Build history of the part. All positions in model axes, mm. Round coordinates to 2 decimals unless told otherwise and drop trailing zeros. Loops run counter-clockwise (first coordinate to the right, second up) from the corner with the lowest first, then second, coordinate; pieces in that order, holes last. Notation, with made-up numbers: (-32.5, 8.25) - (2.5, 8.25) arc R18 cw to (2.5, 20.25) - close; hole circle Ø1 at (59.25, -1). An arc over 180 degrees is marked (long way). Use one line per item in the form item = value. Start each with the question number.
Q1. Saw through at B-B (x = -27). Give the cut face in (y, z).
Q2. Drill centre lines: line 1 (Z direction, x = -26.5, y = 0.8); line 2 (X direction, y = 1.55, z = -35). Where is each one in solid material? Low to high.
Q3. Pin check, flat tips, straight feed: pin 1 (8 mm diameter, centred on x = -1.5, z = -128.5, fed in from -Y); pin 2 (1.5 mm diameter, centred on y = 1, z = -205, fed in from -X); pin 3 (1.5 mm diameter, centred on y = 1.5, z = -79, fed in from -X); pin 4 (1.5 mm diameter, centred on x = -37, y = 2, fed in from -Z). Stop position of each tip, or through.
Q4. Saw through at A-A (z = -177.5). Give the cut face in (x, y).
```python
from build123d import *

# Parameters (mm, degrees)
SKETCH1_W           = 35.65
SKETCH1_H           = 204
BOSS_EXTRUDE1_DEPTH = 3
SKETCH2_W           = 12
SKETCH2_H           = 3
SKETCH2_W_2         = 10
BOSS_EXTRUDE2_DEPTH = 3
ESQUISSE1_W         = 10
ESQUISSE1_H         = 3
BOSS_EXTRU_1_DEPTH  = 3
ESQUISSE2_W         = 10
ESQUISSE2_H         = 3
BOSS_EXTRU_2_DEPTH  = 3


with BuildPart() as part:
    # Sketch1 → Boss-Extrude1 (new body)
    with BuildSketch(Plane(origin=(0, 0, 0), x_dir=(1, 0, 0), z_dir=(0, 1, 0))):
        with Locations((17.825, 102)):
            Rectangle(SKETCH1_W, SKETCH1_H)
    boss_extrude1 = extrude(amount=BOSS_EXTRUDE1_DEPTH)

    # Sketch2 → Boss-Extrude2 (add)
    with BuildSketch(Plane(origin=(35.65, 0, 0), x_dir=(0, 0, -1), z_dir=(1, 0, 0))):
        with Locations((6, 1.5)):
            Rectangle(SKETCH2_W, SKETCH2_H)
        with Locations((27, 1.5)):
            Rectangle(SKETCH2_W_2, SKETCH2_H)
        with Locations((47, 1.5)):
            Rectangle(SKETCH2_W_2, SKETCH2_H)
        with Locations((67, 1.5)):
            Rectangle(SKETCH2_W_2, SKETCH2_H)
        with Locations((87, 1.5)):
            Rectangle(SKETCH2_W_2, SKETCH2_H)
        with Locations((107, 1.5)):
            Rectangle(SKETCH2_W_2, SKETCH2_H)
        with Locations((127, 1.5)):
            Rectangle(SKETCH2_W_2, SKETCH2_H)
        with Locations((147, 1.5)):
            Rectangle(SKETCH2_W_2, SKETCH2_H)
        with Locations((167, 1.5)):
            Rectangle(SKETCH2_W_2, SKETCH2_H)
        with Locations((187, 1.5)):
            Rectangle(SKETCH2_W_2, SKETCH2_H)
    boss_extrude2 = extrude(amount=BOSS_EXTRUDE2_DEPTH)

    # Mirror1: Boss-Extrude1, Boss-Extrude2 across plane
    add(boss_extrude1.mirror(Plane(origin=(0, 0, 0), x_dir=(0, 0, 1), z_dir=(1, 0, 0))))
    add(boss_extrude2.mirror(Plane(origin=(0, 0, 0), x_dir=(0, 0, 1), z_dir=(1, 0, 0))))

    # Esquisse1 → Boss.-Extru.1 (add)
    with BuildSketch(Plane(origin=(0, 0, -204), x_dir=(-1, 0, 0), z_dir=(0, 0, -1))):
        with Locations((-20.65, 1.5)):
            Rectangle(ESQUISSE1_W, ESQUISSE1_H)
        with Locations((-0.65, 1.5)):
            Rectangle(ESQUISSE1_W, ESQUISSE1_H)
        with Locations((19.35, 1.5)):
            Rectangle(ESQUISSE1_W, ESQUISSE1_H)
    extrude(amount=BOSS_EXTRU_1_DEPTH)

    # Esquisse2 → Boss.-Extru.2 (add)
    with BuildSketch(Plane.XY):
        with Locations((-19.35, 1.5)):
            Rectangle(ESQUISSE2_W, ESQUISSE2_H)
        with Locations((0.65, 1.5)):
            Rectangle(ESQUISSE2_W, ESQUISSE2_H)
        with Locations((20.65, 1.5)):
            Rectangle(ESQUISSE2_W, ESQUISSE2_H)
    extrude(amount=BOSS_EXTRU_2_DEPTH)


solid = part.part
```
Report:
q1.outline = (0, -204) - (3, -204) - (3, 0) - (0, 0) - close
q2.line_1 = -204 to 0
q2.line_2 = -35.65 to 35.65
q3.pin_1 = 0
q3.pin_2 = -24.35
q3.pin_3 = -35.65
q3.pin_4 = -192
q4.outline = (-35.65, 0) - (35.65, 0) - (35.65, 3) - (-35.65, 3) - close
